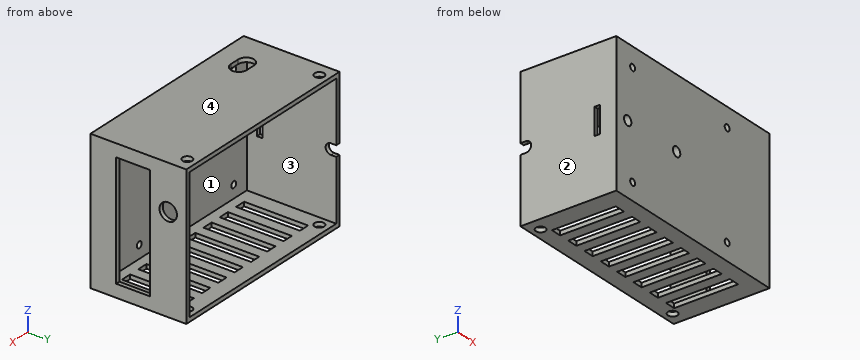
from build123d import *

# Parameters (mm, degrees)
SKETCH1_W           = 90
SKETCH1_H           = 62
BOSS_EXTRUDE1_DEPTH = 3
CUT_EXTRUDE1_REACH  = 56.727
SKETCH2_R           = 1.5
SKETCH3_W           = 94
SKETCH3_H           = 66
SKETCH3_W_2         = 90
SKETCH3_H_2         = 62
BOSS_EXTRUDE2_DEPTH = 45
CUT_EXTRUDE2_REACH  = 109.601
SKETCH4_W           = 12.5
SKETCH4_H           = 2.5
CUT_EXTRUDE3_REACH  = 93.269
CUT_EXTRUDE4_REACH  = 109.601
SKETCH6_W           = 54
SKETCH6_H           = 16
CUT_EXTRUDE5_REACH  = 111.316
SKETCH7_R           = 4.1
SKETCH8_R           = 2.25
CUT_EXTRUDE6_DEPTH  = 93.682252886
CUT_EXTRUDE8_REACH  = 94.682
SKETCH10_W          = 5
SKETCH10_H          = 30
CUT_EXTRUDE9_REACH  = 111.316
CUT_EXTRUDE10_REACH = 74.959
SKETCH12_R          = 2.25


with BuildPart() as part:
    # Sketch1 → Boss-Extrude1 (new body)
    with BuildSketch(Plane(origin=(0, 0, 0), x_dir=(1, 0, 0), z_dir=(0, 1, 0))):
        Rectangle(SKETCH1_W, SKETCH1_H)
    extrude(amount=BOSS_EXTRUDE1_DEPTH)

    # Sketch2 → Cut-Extrude1 (cut, up to next)
    with BuildSketch(Plane(origin=(0, 3, 0), x_dir=(1, 0, 0), z_dir=(0, 1, 0)), mode=Mode.PRIVATE) as cut_extrude1_sk1:
        with Locations(Location((-37, -24, 0), (0, 0, 270))):
            Circle(SKETCH2_R)
    cut_extrude1_tool1 = extrude(cut_extrude1_sk1.sketch, amount=-CUT_EXTRUDE1_REACH, mode=Mode.PRIVATE) & part.part
    # Sketch2 → Cut-Extrude1 (cut, up to next)
    with BuildSketch(Plane(origin=(0, 3, 0), x_dir=(1, 0, 0), z_dir=(0, 1, 0)), mode=Mode.PRIVATE) as cut_extrude1_sk2:
        with Locations(Location((21, -24, 0), (0, 0, 270))):
            Circle(SKETCH2_R)
    cut_extrude1_tool2 = extrude(cut_extrude1_sk2.sketch, amount=-CUT_EXTRUDE1_REACH, mode=Mode.PRIVATE) & part.part
    # Sketch2 → Cut-Extrude1 (cut, up to next)
    with BuildSketch(Plane(origin=(0, 3, 0), x_dir=(1, 0, 0), z_dir=(0, 1, 0)), mode=Mode.PRIVATE) as cut_extrude1_sk3:
        with Locations(Location((21, 25, 0), (0, 0, 270))):
            Circle(SKETCH2_R)
    cut_extrude1_tool3 = extrude(cut_extrude1_sk3.sketch, amount=-CUT_EXTRUDE1_REACH, mode=Mode.PRIVATE) & part.part
    # Sketch2 → Cut-Extrude1 (cut, up to next)
    with BuildSketch(Plane(origin=(0, 3, 0), x_dir=(1, 0, 0), z_dir=(0, 1, 0)), mode=Mode.PRIVATE) as cut_extrude1_sk4:
        with Locations(Location((-37, 25, 0), (0, 0, 270))):
            Circle(SKETCH2_R)
    cut_extrude1_tool4 = extrude(cut_extrude1_sk4.sketch, amount=-CUT_EXTRUDE1_REACH, mode=Mode.PRIVATE) & part.part
    add(cut_extrude1_tool1.solids().sort_by_distance((-37, 3, 24))[0], mode=Mode.SUBTRACT)
    add(cut_extrude1_tool2.solids().sort_by_distance((21, 3, 24))[0], mode=Mode.SUBTRACT)
    add(cut_extrude1_tool3.solids().sort_by_distance((21, 3, -25))[0], mode=Mode.SUBTRACT)
    add(cut_extrude1_tool4.solids().sort_by_distance((-37, 3, -25))[0], mode=Mode.SUBTRACT)

    # Sketch3 → Boss-Extrude2 (add)
    with BuildSketch(Plane(origin=(0, 0, 0), x_dir=(1, 0, 0), z_dir=(0, 1, 0))):
        Rectangle(SKETCH3_W, SKETCH3_H)
        Rectangle(SKETCH3_W_2, SKETCH3_H_2, mode=Mode.SUBTRACT)
    extrude(amount=BOSS_EXTRUDE2_DEPTH)

    # Sketch4 → Cut-Extrude2 (cut, up to next)
    with BuildSketch(Plane(origin=(-45, 0, 0), x_dir=(0, 0, -1), z_dir=(1, 0, 0)), mode=Mode.PRIVATE) as cut_extrude2_sk1:
        with Locations((0, 9)):
            Rectangle(SKETCH4_W, SKETCH4_H)
    cut_extrude2_tool1 = extrude(cut_extrude2_sk1.sketch, amount=-CUT_EXTRUDE2_REACH, mode=Mode.PRIVATE) & part.part
    add(cut_extrude2_tool1.solids().sort_by_distance((-45, 9, 0))[0], mode=Mode.SUBTRACT)

    # Sketch5 → Cut-Extrude3 (cut, up to next)
    with BuildSketch(Plane(origin=(0, 0, 31), x_dir=(-1, 0, 0), z_dir=(0, 0, -1)), mode=Mode.PRIVATE) as cut_extrude3_sk1:
        with BuildLine():
            Line((31.55, 9.25), (27.05, 9.25))
            ThreePointArc((27.05, 9.25), (23.3, 13), (27.05, 16.75))
            Line((27.05, 16.75), (31.55, 16.75))
            ThreePointArc((31.55, 16.75), (35.3, 13), (31.55, 9.25))
        make_face()
    cut_extrude3_tool1 = extrude(cut_extrude3_sk1.sketch, amount=-CUT_EXTRUDE3_REACH, mode=Mode.PRIVATE) & part.part
    add(cut_extrude3_tool1.solids().sort_by_distance((-29.3, 13, 31))[0], mode=Mode.SUBTRACT)

    # Sketch6 → Cut-Extrude4 (cut, up to next)
    with BuildSketch(Plane.ZY.offset(-45), mode=Mode.PRIVATE) as cut_extrude4_sk1:
        with Locations((0, 20)):
            Rectangle(SKETCH6_W, SKETCH6_H)
    cut_extrude4_tool1 = extrude(cut_extrude4_sk1.sketch, amount=-CUT_EXTRUDE4_REACH, mode=Mode.PRIVATE) & part.part
    add(cut_extrude4_tool1.solids().sort_by_distance((45, 20, 0))[0], mode=Mode.SUBTRACT)

    # Sketch7 → Cut-Extrude5 (cut, up to next)
    with BuildSketch(Plane(origin=(47, 0, 0), x_dir=(0, 0, -1), z_dir=(1, 0, 0)), mode=Mode.PRIVATE) as cut_extrude5_sk1:
        with Locations((-12, 36.5)):
            Circle(SKETCH7_R)
    cut_extrude5_tool1 = extrude(cut_extrude5_sk1.sketch, amount=-CUT_EXTRUDE5_REACH, mode=Mode.PRIVATE) & part.part
    add(cut_extrude5_tool1.solids().sort_by_distance((47, 36.5, 12))[0], mode=Mode.SUBTRACT)

    # Sketch8 → Cut-Extrude6 (cut, through all)
    with BuildSketch(Plane.XY.offset(33)):
        with Locations((-40.5, 40.5)):
            Circle(SKETCH8_R)
        with Locations(Location((40.5, 40.5, 0), (0, 0, 180))):
            Circle(SKETCH8_R)
    extrude(amount=-CUT_EXTRUDE6_DEPTH, mode=Mode.SUBTRACT)

    # Sketch10 → Cut-Extrude8 (cut, up to next)
    with BuildSketch(Plane(origin=(0, 0, -33), x_dir=(-1, 0, 0), z_dir=(0, 0, -1)), mode=Mode.PRIVATE) as cut_extrude8_sk1:
        with Locations((15, 22.5)):
            Rectangle(SKETCH10_W, SKETCH10_H)
    cut_extrude8_tool1 = extrude(cut_extrude8_sk1.sketch, amount=-CUT_EXTRUDE8_REACH, mode=Mode.PRIVATE) & part.part
    # Sketch10 → Cut-Extrude8 (cut, up to next)
    with BuildSketch(Plane(origin=(0, 0, -33), x_dir=(-1, 0, 0), z_dir=(0, 0, -1)), mode=Mode.PRIVATE) as cut_extrude8_sk2:
        with Locations((5, 22.5)):
            Rectangle(SKETCH10_W, SKETCH10_H)
    cut_extrude8_tool2 = extrude(cut_extrude8_sk2.sketch, amount=-CUT_EXTRUDE8_REACH, mode=Mode.PRIVATE) & part.part
    # Sketch10 → Cut-Extrude8 (cut, up to next)
    with BuildSketch(Plane(origin=(0, 0, -33), x_dir=(-1, 0, 0), z_dir=(0, 0, -1)), mode=Mode.PRIVATE) as cut_extrude8_sk3:
        with Locations((25, 22.5)):
            Rectangle(SKETCH10_W, SKETCH10_H)
    cut_extrude8_tool3 = extrude(cut_extrude8_sk3.sketch, amount=-CUT_EXTRUDE8_REACH, mode=Mode.PRIVATE) & part.part
    # Sketch10 → Cut-Extrude8 (cut, up to next)
    with BuildSketch(Plane(origin=(0, 0, -33), x_dir=(-1, 0, 0), z_dir=(0, 0, -1)), mode=Mode.PRIVATE) as cut_extrude8_sk4:
        with Locations((35, 22.5)):
            Rectangle(SKETCH10_W, SKETCH10_H)
    cut_extrude8_tool4 = extrude(cut_extrude8_sk4.sketch, amount=-CUT_EXTRUDE8_REACH, mode=Mode.PRIVATE) & part.part
    # Sketch10 → Cut-Extrude8 (cut, up to next)
    with BuildSketch(Plane(origin=(0, 0, -33), x_dir=(-1, 0, 0), z_dir=(0, 0, -1)), mode=Mode.PRIVATE) as cut_extrude8_sk5:
        with Locations((-5, 22.5)):
            Rectangle(SKETCH10_W, SKETCH10_H)
    cut_extrude8_tool5 = extrude(cut_extrude8_sk5.sketch, amount=-CUT_EXTRUDE8_REACH, mode=Mode.PRIVATE) & part.part
    # Sketch10 → Cut-Extrude8 (cut, up to next)
    with BuildSketch(Plane(origin=(0, 0, -33), x_dir=(-1, 0, 0), z_dir=(0, 0, -1)), mode=Mode.PRIVATE) as cut_extrude8_sk6:
        with Locations((-15, 22.5)):
            Rectangle(SKETCH10_W, SKETCH10_H)
    cut_extrude8_tool6 = extrude(cut_extrude8_sk6.sketch, amount=-CUT_EXTRUDE8_REACH, mode=Mode.PRIVATE) & part.part
    # Sketch10 → Cut-Extrude8 (cut, up to next)
    with BuildSketch(Plane(origin=(0, 0, -33), x_dir=(-1, 0, 0), z_dir=(0, 0, -1)), mode=Mode.PRIVATE) as cut_extrude8_sk7:
        with Locations((-25, 22.5)):
            Rectangle(SKETCH10_W, SKETCH10_H)
    cut_extrude8_tool7 = extrude(cut_extrude8_sk7.sketch, amount=-CUT_EXTRUDE8_REACH, mode=Mode.PRIVATE) & part.part
    # Sketch10 → Cut-Extrude8 (cut, up to next)
    with BuildSketch(Plane(origin=(0, 0, -33), x_dir=(-1, 0, 0), z_dir=(0, 0, -1)), mode=Mode.PRIVATE) as cut_extrude8_sk8:
        with Locations((-35, 22.5)):
            Rectangle(SKETCH10_W, SKETCH10_H)
    cut_extrude8_tool8 = extrude(cut_extrude8_sk8.sketch, amount=-CUT_EXTRUDE8_REACH, mode=Mode.PRIVATE) & part.part
    add(cut_extrude8_tool1.solids().sort_by_distance((-15, 22.5, -33))[0], mode=Mode.SUBTRACT)
    add(cut_extrude8_tool2.solids().sort_by_distance((-5, 22.5, -33))[0], mode=Mode.SUBTRACT)
    add(cut_extrude8_tool3.solids().sort_by_distance((-25, 22.5, -33))[0], mode=Mode.SUBTRACT)
    add(cut_extrude8_tool4.solids().sort_by_distance((-35, 22.5, -33))[0], mode=Mode.SUBTRACT)
    add(cut_extrude8_tool5.solids().sort_by_distance((5, 22.5, -33))[0], mode=Mode.SUBTRACT)
    add(cut_extrude8_tool6.solids().sort_by_distance((15, 22.5, -33))[0], mode=Mode.SUBTRACT)
    add(cut_extrude8_tool7.solids().sort_by_distance((25, 22.5, -33))[0], mode=Mode.SUBTRACT)
    add(cut_extrude8_tool8.solids().sort_by_distance((35, 22.5, -33))[0], mode=Mode.SUBTRACT)

    # Sketch11 → Cut-Extrude9 (cut, up to next)
    with BuildSketch(Plane.ZY.offset(47), mode=Mode.PRIVATE) as cut_extrude9_sk1:
        with BuildLine():
            Line((2.5, 47.5), (2.5, 42.5))
            ThreePointArc((2.5, 42.5), (0, 40), (-2.5, 42.5))
            Line((-2.5, 42.5), (-2.5, 47.5))
            ThreePointArc((-2.5, 47.5), (0, 50), (2.5, 47.5))
        make_face()
    cut_extrude9_tool1 = extrude(cut_extrude9_sk1.sketch, amount=-CUT_EXTRUDE9_REACH, mode=Mode.PRIVATE) & part.part
    add(cut_extrude9_tool1.solids().sort_by_distance((-47, 45, 0))[0], mode=Mode.SUBTRACT)

    # Sketch12 → Cut-Extrude10 (cut, up to next)
    with BuildSketch(Plane.XZ, mode=Mode.PRIVATE) as cut_extrude10_sk1:
        with Locations(Location((-40, 0, 0), (0, 0, 270))):
            Circle(SKETCH12_R)
    cut_extrude10_tool1 = extrude(cut_extrude10_sk1.sketch, amount=-CUT_EXTRUDE10_REACH, mode=Mode.PRIVATE) & part.part
    # Sketch12 → Cut-Extrude10 (cut, up to next)
    with BuildSketch(Plane.XZ, mode=Mode.PRIVATE) as cut_extrude10_sk2:
        with Locations(Location((-10, 0, 0), (0, 0, 270))):
            Circle(SKETCH12_R)
    cut_extrude10_tool2 = extrude(cut_extrude10_sk2.sketch, amount=-CUT_EXTRUDE10_REACH, mode=Mode.PRIVATE) & part.part
    add(cut_extrude10_tool1.solids().sort_by_distance((-40, 0, 0))[0], mode=Mode.SUBTRACT)
    add(cut_extrude10_tool2.solids().sort_by_distance((-10, 0, 0))[0], mode=Mode.SUBTRACT)


solid = part.part
For this review, take the finished solid that the model builds, in its own axes (mm). Face numbers are marked on the shaded views. Give positions to 0.01 mm unless a question says otherwise; leave off trailing zeros. Loops run counter-clockwise (first coordinate to the right, second up) from the corner with the lowest first, then second, coordinate; pieces in that order, holes last. Notation, with made-up numbers: M 4.5,45 L 50.5,45 A35 cw 50.5,78 Z; hole C 70.5,-4.5 d7. An arc over 180 degrees is marked long. Put each result on its own line as item: value. Start each with the question number.
(1) Wall thickness on L1, parallel to X at y = 0.7, z = 0; L2, parallel to X at y = 1, z = 24; L3, parallel to Z at x = -1, y = 28.5: over which ranges is each line inside the solid? List them lowest first.
(2) Add section D-D, the plane y = 5. Write out the cut boundary in (x, z).
(3) Add section A-A, the plane z = -12. Write out the cut boundary in (x, y), then the cut area to 3 significant figures.
(4) The part is to be moulded in two halves that separate along X. For the marked faces 1, 2, 3 and 4, say which applies: +X half, -X half, draft (parallel to the pull), parting line (faces both ways), or undercut.
(5) Add section C-C, the plane z = 24. Write out the cut boundary in (x, y), then the cut area to 3 significant figures.
(6) For pin 1 (3 mm diameter, centred on y = 15.5, z = 19, fed in from +X); pin 2 (2.5 mm diameter, centred on x = -37, z = 24, fed in from -Y), all flat-tipped, find the tip position at first contact; note any pin that passes through.
(7) Add section B-B, the plane x = 40.5. Write out the cut boundary in (y, z), then the cut area to 3 significant figures.
Result:
1. L1: x = -47 to -42.25, -37.75 to -12.25, -7.75 to 47
1. L2: x = -47 to -38.5, -35.5 to 19.5, 22.5 to 47
1. L3: z = -33 to -31, 31 to 33
2. outline: M -47,-33 L 47,-33 L 47,33 L -47,33 Z; hole M -45,-31 L 45,-31 L 45,31 L -45,31 Z
3. outline: M -47,0 L 47,0 L 47,12 L 45,12 L 45,3 L -45,3 L -45,45 L -47,45 Z; M 45,28 L 47,28 L 47,45 L 45,45 Z
3. area: 418 mm^2
4. face 1: undercut
4. face 2: -X half
4. face 3: undercut
4. face 4: draft
5. outline: M -47,0 L -38.5,0 L -38.5,3 L -45,3 L -45,45 L -47,45 Z; M -35.5,0 L 19.5,0 L 19.5,3 L -35.5,3 Z; M 22.5,0 L 47,0 L 47,12 L 45,12 L 45,3 L 22.5,3 Z; M 45,28 L 47,28 L 47,45 L 45,45 Z
5. area: 400 mm^2
6. pin 1: stops at x = -45
6. pin 2: passes through
7. outline: M 0,-33 L 38.25,-33 L 38.25,-31 L 3,-31 L 3,31 L 38.25,31 L 38.25,33 L 0,33 Z; M 42.75,-33 L 45,-33 L 45,-31 L 42.75,-31 Z; M 42.75,31 L 45,31 L 45,33 L 42.75,33 Z
7. area: 348 mm^2
